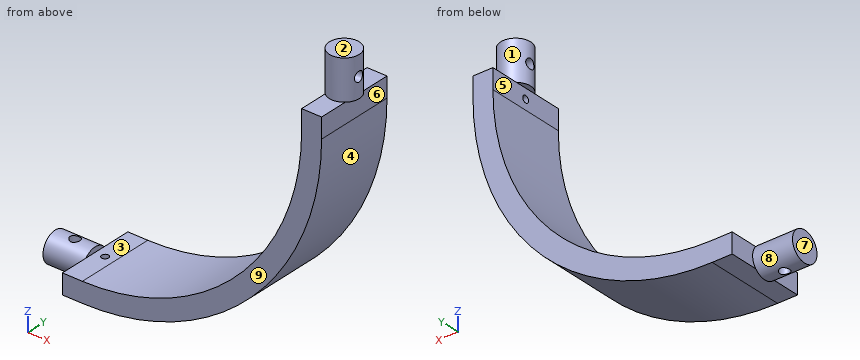
```python
from build123d import *

# Parameters (mm, degrees)
BOSS_EXTRUDE1_DEPTH = 25.4
SKETCH2_W           = 12.7
SKETCH2_H           = 50.8
BOSS_EXTRUDE2_DEPTH = 12.7
SKETCH3_W           = 12.7
SKETCH3_H           = 50.8
BOSS_EXTRUDE3_DEPTH = 12.7
SKETCH4_R           = 9.525
BOSS_EXTRUDE4_DEPTH = 25.4
SKETCH5_R           = 3.175
CUT_EXTRUDE1_DEPTH  = 19.05
SKETCH6_R           = 9.525
BOSS_EXTRUDE5_DEPTH = 25.4
SKETCH7_R           = 3.175
CUT_EXTRUDE2_DEPTH  = 19.05
SKETCH8_R           = 2.2225
CUT_EXTRUDE3_DEPTH  = 11.43
SKETCH9_R           = 2.2225
CUT_EXTRUDE4_DEPTH  = 11.43


with BuildPart() as part:
    # Sketch1 → Boss-Extrude1 (new, symmetric)
    with BuildSketch(Plane(origin=(0, 0, 0), x_dir=(1, 0, 0), z_dir=(0, 1, 0))):
        with BuildLine():
            Line((0, 152.4), (0, 139.7))
            ThreePointArc((0, 139.7), (98.782817332, 98.782817332), (139.7, 0))
            Line((139.7, 0), (152.4, 0))
            ThreePointArc((152.4, 0), (107.763073453, 107.763073453), (0, 152.4))
        make_face()
    extrude(amount=BOSS_EXTRUDE1_DEPTH, both=True)

    # Sketch2 → Boss-Extrude2 (add)
    with BuildSketch(Plane.ZY):
        with Locations((-146.05, 0)):
            Rectangle(SKETCH2_W, SKETCH2_H)
    extrude(amount=BOSS_EXTRUDE2_DEPTH)

    # Sketch3 → Boss-Extrude3 (add)
    with BuildSketch(Plane.XY):
        with Locations((146.05, 0)):
            Rectangle(SKETCH3_W, SKETCH3_H)
    extrude(amount=BOSS_EXTRUDE3_DEPTH)

    # Sketch4 → Boss-Extrude4 (add)
    with BuildSketch(Plane.ZY.offset(12.7)):
        with Locations(Location((-146.05, 0, 0), (0, 0, 131.810314896))):
            Circle(SKETCH4_R)
    extrude(amount=BOSS_EXTRUDE4_DEPTH)

    # Sketch5 → Cut-Extrude1 (cut, symmetric)
    with BuildSketch(Plane.XY.offset(-139.7)):
        with Locations((-25.4, 0)):
            Circle(SKETCH5_R)
    extrude(amount=CUT_EXTRUDE1_DEPTH, both=True, mode=Mode.SUBTRACT)

    # Sketch6 → Boss-Extrude5 (add)
    with BuildSketch(Plane.XY.offset(12.7)):
        with Locations(Location((146.05, 0, 0), (0, 0, 131.810314896))):
            Circle(SKETCH6_R)
    extrude(amount=BOSS_EXTRUDE5_DEPTH)

    # Sketch7 → Cut-Extrude2 (cut, symmetric)
    with BuildSketch(Plane.ZY.offset(-139.7)):
        with Locations((25.4, 0)):
            Circle(SKETCH7_R)
    extrude(amount=CUT_EXTRUDE2_DEPTH, both=True, mode=Mode.SUBTRACT)

    # Sketch8 → Cut-Extrude3 (cut)
    with BuildSketch(Plane.XY.offset(-139.7)):
        with Locations((-6.35, 0)):
            Circle(SKETCH8_R)
    extrude(amount=-CUT_EXTRUDE3_DEPTH, mode=Mode.SUBTRACT)

    # Sketch9 → Cut-Extrude4 (cut)
    with BuildSketch(Plane.ZY.offset(-139.7)):
        with Locations((6.35, 0)):
            Circle(SKETCH9_R)
    extrude(amount=-CUT_EXTRUDE4_DEPTH, mode=Mode.SUBTRACT)


solid = part.part
```
For this review, take the finished solid that the model builds, in its own axes (mm). Face numbers are marked on the shaded views. A direction names the side the tool comes from. Coordinates: 2 decimals unless noted, no trailing zeros. Loops run counter-clockwise (first coordinate to the right, second up) from the corner with the lowest first, then second, coordinate; pieces in that order, holes last. Notation, with made-up numbers: (21, 6.25) -> (25, 6.25) arc R23 ccw to (25, 34.25) -> close; hole circle Ø7 at (56.25, -4.5). An arc over 180 degrees is marked (long way). Return JSON: item names as keys, results as strings. Group by question number.
(1) Consider section A-A, the plane y = 21. Give the boundary of the cut face in (x, z), plus the area to 3 significant figures.
(2) Consider section B-B, the plane x = 146.05. Count the separate pieces of the cut face and the enclosed holes in it, plus the area to 3 significant figures.
(3) For pin 1 Ø14 at (y, z) = (16, -148.5) entering from -X; pin 2 Ø1 at (y, z) = (2.5, -153.5) entering from +X; pin 3 Ø4 at (x, y) = (146.5, -18) entering from +Z; pin 4 Ø6 at (y, z) = (0, 6.35) entering from -X, all flat-tipped, find the tip position at first contact; note any pin that passes through.
(4) Mouldability with a two-part tool opening along X and no side actions: class the marked faces 1, 2, 3 and 4 as pulls with the +X half, pulls with the -X half, needs draft (parallel to the pull), parting line crosses it, or undercut.
(5) Consider section D-D, the plane x = -25.4. Give the boundary of the cut face in (y, z) (3 decimals), plus the area to 3 significant figures.
(6) To check wall thickness, follow L1, parallel to Y at x = -6.35, z = -145.5; L2, parallel to Y at x = 145.75, z = 25.4 (3 decimals); L3, parallel to Z at x = -6, y = 6. State the ranges of each line that lie inside material, in increasing order.
(7) Tool access review of the marked faces 5, 6, 7, 8 and 9: name each direction out of +Z, -Z, +X, -X, +Y, -Y from which nothing blocks a thin tool from reaching the whole face with its end or side.
Results below:
{
 "1": {"outline": "(-12.7, -152.4) -> (0, -152.4) arc R152.4 ccw to (152.4, 0) -> (152.4, 12.7) -> (139.7, 12.7) -> (139.7, 0) arc R139.7 cw to (0, -139.7) -> (-12.7, -139.7) -> close", "area": "3,240 mm2"},
 "2": {"separate pieces": "1", "enclosed holes": "2", "area": "3,290 mm2"},
 "3": {"pin 1": "stops at x = -38.1", "pin 2": "stops at x = -12.7", "pin 3": "stops at z = 12.7", "pin 4": "stops at x = 139.7"},
 "4": {"face 1": "parting line crosses it", "face 2": "needs draft", "face 3": "undercut", "face 4": "pulls with the +X half"},
 "5": {"outline": "(-3.175, -155.03) -> (-3.175, -137.07) arc R9.525 ccw to start; (3.175, -155.03) arc R9.525 ccw to (3.175, -137.07) -> close", "area": "166 mm2"},
 "6": {"L1": "y = -25.4 to -2.22, 2.22 to 25.4", "L2": "y = -9.52 to -3.175, 3.175 to 9.52", "L3": "z = -152.4 to -139.7"},
 "7": {"face 5": "-X, +Y, -Y", "face 6": "-Z, +X, +Y, -Y", "face 7": "+Z, -Z, -X, +Y, -Y", "face 8": "-X", "face 9": "+Z, -Z, +X, -X, -Y"}
}
